For this review, use the dimensioned drawing (mm, ordinates from the lowest corner) and the shaded views. A direction names the side the tool comes from. Coordinates: 2 decimals unless noted, no trailing zeros. Write each loop counter-clockwise with the first axis right and the second up, starting at its lowest first coordinate (ties: lowest second). Pieces come first, ordered by that corner, then holes.
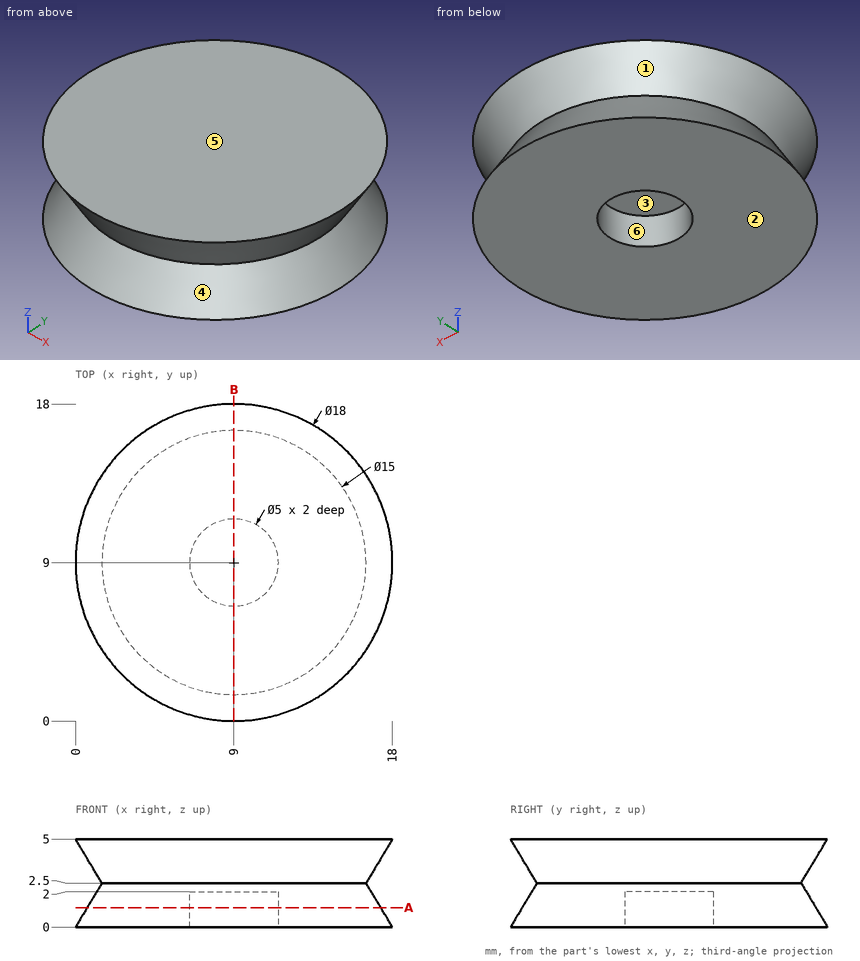
Item 1: Take a section at B-B, the plane x = 9. Write out the cut boundary in (y, z), plus the area to 3 significant figures.
Solved:
outline: (0, 0) - (6.5, 0) - (6.5, 2) - (11.5, 2) - (11.5, 0) - (18, 0) - (16.5, 2.5) - (18, 5) - (0, 5) - (1.5, 2.5) - close
area: 72.5 mm2
Item 2: Machinability: for the marked faces 1 and 2, which of the approach directions +Z, -Z, +X, -X, +Y, -Y give a long, thin tool a straight path to every point of the face, cutting with its end or side? Answer none if there is none.
Solved:
face 1: none
face 2: -Z, +X, -X, +Y, -Y
Item 3: Take a section at A-A, the plane z = 1.1. Write out the cut boundary in (x, y).
Solved:
outline: circle Ø16.68 at (9, 9); hole circle Ø5 at (9, 9)
Item 4: To check wall thickness, follow line 1 along X through (y, z) = (7.25, 0.4); line 2 along Y through (x, z) = (9, 1.45); line 3 along Z through (x, y) = (8.5, 1). State the ranges of each line that lie inside material, in increasing order.
Solved:
line 1: x = 0.42 to 7.21, 10.79 to 17.58
line 2: y = 0.87 to 6.5, 11.5 to 17.13
line 3: z = 0 to 1.64, 3.36 to 5
Item 5: Mouldability with a two-part tool opening along X and no side actions: class the marked faces 3, 4, 5 and 6 as pulls with the +X half, pulls with the -X half, needs draft (parallel to the pull), parting line crosses it, or undercut.
Solved:
face 3: undercut
face 4: parting line crosses it
face 5: needs draft
face 6: undercut
